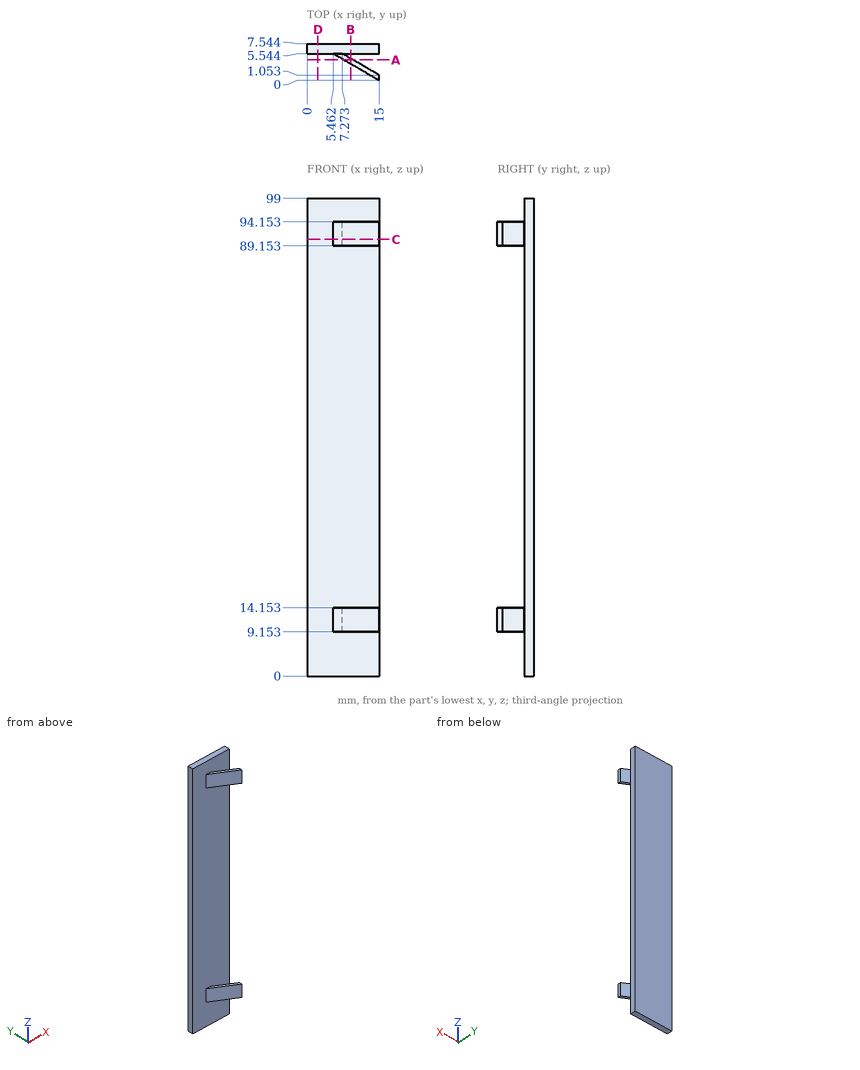
Design review of the part shown in the three views and the two pictorial views. Dimensions are in mm from the part's minimum x, y and z. Round coordinates to 2 decimals unless told otherwise and drop trailing zeros. Write each loop counter-clockwise with the first axis right and the second up, starting at its lowest first coordinate (ties: lowest second). Pieces come first, ordered by that corner, then holes. Notation, with made-up numbers: M 59,15.25 L 99,15.25 A27 ccw 99,35.25 Z; hole C -7.75,-6 d1. An arc over 180 degrees is marked long. One line per item, written item: value. Start each with the question number.
1. Clearance check with flat-ended pins moving along their axes: P1, Ø7.5, axis at x = 6.5, z = 72, coming from the -Y side; P2, Ø1.5, axis at x = 10.5, y = 1, coming from the +Z side (3 decimals); P3, Ø3, axis at x = 13, y = 2, coming from the -Z side; P4, Ø4.5, axis at x = 10.5, y = 2, coming from the +Z side. State where each tip first meets the part, or that it passes through.
2. Take a section at A-A on y = 4.25. State the section outline as (x, z) points, then the cut area to 3 significant figures.
3. Take a section at B-B on x = 9. State the section outline as (y, z) points.
4. To check wall thickness, follow probe 1 along Y at (x, z) = (4.25, 18); probe 2 along Y at (x, z) = (11, 92.5) (1 decimal); probe 3 along Y at (x, z) = (6.25, 11) (1 decimal). State the ranges of each line that lie inside material, in increasing order. Write a range as from..to.
5. Take a section at C-C on z = 90.5. State the section outline as (x, y) points.
6. Take a section at D-D on x = 2.25. State the section outline as (y, z) points.
Computed:
1. P1: stops at y = 5.54
1. P2: passes through
1. P3: stops at z = 9.15
1. P4: stops at z = 94.15
2. outline: M 7.69,9.15 L 9.5,9.15 L 9.5,14.15 L 7.69,14.15 Z; M 7.69,89.15 L 9.5,89.15 L 9.5,94.15 L 7.69,94.15 Z
2. area: 18.1 mm²
3. outline: M 3.49,9.15 L 4.54,9.15 L 4.54,14.15 L 3.49,14.15 Z; M 3.49,89.15 L 4.54,89.15 L 4.54,94.15 L 3.49,94.15 Z; M 5.54,0 L 7.54,0 L 7.54,99 L 5.54,99 Z
4. probe 1: y = 5.54..7.54
4. probe 2: y = 2.3..3.4, 5.5..7.5
4. probe 3: y = 5.1..7.5
5. outline: M 0,5.54 L 5.46,5.54 L 15,0 L 15,1.05 L 7.27,5.54 L 15,5.54 L 15,7.54 L 0,7.54 Z
6. outline: M 5.54,0 L 7.54,0 L 7.54,99 L 5.54,99 Z
